```python
from build123d import *

# Parameters (mm, degrees)
F0_R     = 20
F1_DEPTH = 200
F2_R     = 51.8547175937
F2_R_2   = 20
F3_DEPTH = 25
F4_SIZE  = 5
F6_START = -25
F5_R     = 7.1981981043
F6_DEPTH = 26.8557175937


with BuildPart() as f1:
    # F0 (on Front) → F1 (new body)
    with BuildSketch(Plane.XZ):
        Circle(F0_R)
    extrude(amount=F1_DEPTH)

    # F2 (on face) → F3 (join)
    with BuildSketch(Plane.XZ.offset(200)):
        Circle(F2_R)
        Circle(F2_R_2, mode=Mode.SUBTRACT)
        Circle(F2_R)
    extrude(amount=F3_DEPTH)

    # F4
    f4_edges = [f1.edges().sort_by_distance(p)[0] for p in [
        (-51.854718, -225, 0),
        (-51.854718, -200, 0),
        (-20, 0, 0),
    ]]
    chamfer(f4_edges, length=F4_SIZE)

    # F5 (on Top) → F6 (cut)
    with BuildSketch(Plane.XY.offset(F6_START)):
        with Locations((0, -18.5775626451)):
            Circle(F5_R)
    extrude(amount=-F6_DEPTH, mode=Mode.SUBTRACT)


solid = f1.part
```
Model file for the job. Use its own axes, mm. A direction names the side the tool comes from. Give positions to 0.01 mm unless a question says otherwise; leave off trailing zeros. Order: outer loops, then holes, each group sorted by start corner. A loop starts at its lowest first (then second) coordinate and runs counter-clockwise, first axis right, second up.
1) Saw through at C-C, the plane y = -51. Write the cut outline in (x, z), then the cut area to 3 significant figures.
2) Saw through at B-B, the plane z = 0. Write the cut outline in (x, y).
3) Wall check: probe 1 along Y at (x, z) = (-8.5, -20); probe 2 along X at (y, z) = (-121, 0.5). Give the ranges that are in metal, low to high.
4) 3-axis set-ups, long thin cutter, end or side, ignore diameter. For faces 1 (the cylindrical face through (-4.336, -101.135, -19.524)), 2 (the conical face through (43.506, -224.757, -18.039)): which of +Z, -Z, +X, -X, +Y, -Y reach the whole face in a straight line?
5) Saw through at A-A, the plane x = 0. Write the cut outline in (y, z).
6) Pin check, flat tips, straight feed: pin 1 (1 mm diameter, centred on x = 16, z = -33, fed in from +Y); pin 2 (1 mm diameter, centred on x = 20, z = -2.5, fed in from +Y); pin 3 (8 mm diameter, centred on x = -1, y = -119.5, fed in from +Z); pin 4 (8 mm diameter, centred on x = 26, y = -84, fed in from +Z). Stop position of each tip, or through.
Computed:
1. outline: circle Ø40 at (0, 0)
1. area: 1,260 mm2
2. outline: (-51.85, -220) - (-46.85, -225) - (46.85, -225) - (51.85, -220) - (51.85, -205) - (46.85, -200) - (20, -200) - (20, -5) - (15, 0) - (-15, 0) - (-20, -5) - (-20, -200) - (-46.85, -200) - (-51.85, -205) - close
3. probe 1: y = -225 to -200
3. probe 2: x = -19.99 to 19.99
4. face 1: +Y
4. face 2: -Y
5. outline: (-225, -46.85) - (-220, -51.85) - (-205, -51.85) - (-200, -46.85) - (-200, -20) - (-5, -20) - (0, -15) - (0, 15) - (-5, 20) - (-200, 20) - (-200, 46.85) - (-205, 51.85) - (-220, 51.85) - (-225, 46.85) - close
6. pin 1: stops at y = -200
6. pin 2: stops at y = -4.66
6. pin 3: stops at z = 20
6. pin 4: passes through
